from build123d import *

# Parameters (mm, degrees)
SKETCH1_R           = 25
BOSS_EXTRUDE1_DEPTH = 3.5
SKETCH2_R           = 8.05
SKETCH2_R_2         = 6.05
BOSS_EXTRUDE2_DEPTH = 5.5
SKETCH3_R           = 6.15
BOSS_EXTRUDE3_DEPTH = 3


with BuildPart() as part:
    # Sketch1 → Boss-Extrude1 (new body)
    with BuildSketch(Plane(origin=(0, 0, 0), x_dir=(1, 0, 0), z_dir=(0, 1, 0))):
        with Locations(Location((0, 0, 0), (0, 0, 270))):
            Circle(SKETCH1_R)
    extrude(amount=BOSS_EXTRUDE1_DEPTH)

    # Sketch2 → Boss-Extrude2 (add)
    with BuildSketch(Plane(origin=(0, 3.5, 0), x_dir=(1, 0, 0), z_dir=(0, 1, 0))):
        with Locations(Location((0, 0, 0), (0, 0, 270))):
            Circle(SKETCH2_R)
        with Locations(Location((0, 0, 0), (0, 0, 270))):
            Circle(SKETCH2_R_2, mode=Mode.SUBTRACT)
    extrude(amount=BOSS_EXTRUDE2_DEPTH)

    # Sketch3 → Boss-Extrude3 (add)
    with BuildSketch(Plane(origin=(0, 3.5, 0), x_dir=(1, 0, 0), z_dir=(0, 1, 0))):
        Circle(SKETCH3_R)
    extrude(amount=BOSS_EXTRUDE3_DEPTH)


solid = part.part
Source: CAD feature listing. Evaluate the final solid. Frame: model axes, mm. A direction names the side the tool comes from. Round coordinates to 2 decimals unless told otherwise and drop trailing zeros. Order: outer loops, then holes, each group sorted by start corner. A loop starts at its lowest first (then second) coordinate and runs counter-clockwise, first axis right, second up. Notation, with made-up numbers: (68.5, 0.25) - (117.5, 0.25) arc R10 cw to (117.5, 15.25) - close; hole circle Ø4 at (-15.75, -24). An arc over 180 degrees is marked (long way). Use a Markdown table: item, result. Add a question column.
1. Set-up query: faces 1 (the flat face through (6, 3.5, -6)), 2 (the flat face through (0, 0, 0)). Return all of +Z, -Z, +X, -X, +Y, -Y with unobstructed straight access to the full face (end or side cutting, diameter ignored); none if empty.
2. Section query D-D (y = 7.5). Return the cut outline in (x, z), then the cut area to 3 significant figures.
3. Section query B-B (x = 0). Return the cut outline in (y, z).
4. Section query C-C (y = 4.5). Return the cut outline in (x, z), then the cut area to 3 significant figures.
5. First-contact query: pin 1 (5 mm diameter, centred on y = 7, z = -15.5, fed in from +X); pin 2 (5 mm diameter, centred on x = -17, z = 14.5, fed in from +Y); pin 3 (3 mm diameter, centred on x = 17.5, y = 2.5, fed in from +Z); pin 4 (3.5 mm diameter, centred on x = -2, z = 1.5, fed in from +Y). Flat tips, straight axial feed; report the tip coordinate or a pass-through.
6. Mould query, pull axis Z, two halves, no side actions, for faces 3 (the cylindrical face through (7.509, 1.726, 23.846)), 4 (the cylindrical face through (1.82, 7.73, 5.77)), 5 (the flat face through (0, 6.5, 0)), 6 (the flat face through (6, 9, -2)). Classes: +Z half, -Z half, draft (parallel to the pull), parting line (faces both ways), or undercut.
7. Line query: probe 1 along X at (y, z) = (7.5, 0); probe 2 along Y at (x, z) = (16, -5.5); probe 3 along Y at (x, z) = (4, -3). Output: solid intervals per line, ascending.
8. Section query A-A (z = 0). Return the cut outline in (x, y), then the cut area to 3 significant figures.
Derived:
| question | item | result |
|---|---|---|
| 1 | face 1 | +Y |
| 1 | face 2 | +Z, -Z, +X, -X, -Y |
| 2 | outline | circle Ø16.1 at (0, 0); hole circle Ø12.1 at (0, 0) |
| 2 | area | 88.6 mm2 |
| 3 | outline | (0, -25) - (3.5, -25) - (3.5, -8.05) - (9, -8.05) - (9, -6.05) - (6.5, -6.05) - (6.5, 6.05) - (9, 6.05) - (9, 8.05) - (3.5, 8.05) - (3.5, 25) - (0, 25) - close |
| 4 | outline | circle Ø16.1 at (0, 0) |
| 4 | area | 204 mm2 |
| 5 | pin 1 | through |
| 5 | pin 2 | y = 3.5 |
| 5 | pin 3 | z = 19.21 |
| 5 | pin 4 | y = 6.5 |
| 6 | face 3 | parting line |
| 6 | face 4 | undercut |
| 6 | face 5 | undercut |
| 6 | face 6 | draft |
| 7 | probe 1 | -8.05 to -6.05, 6.05 to 8.05 |
| 7 | probe 2 | 0 to 3.5 |
| 7 | probe 3 | 0 to 6.5 |
| 8 | outline | (-25, 0) - (25, 0) - (25, 3.5) - (8.05, 3.5) - (8.05, 9) - (6.05, 9) - (6.05, 6.5) - (-6.05, 6.5) - (-6.05, 9) - (-8.05, 9) - (-8.05, 3.5) - (-25, 3.5) - close |
| 8 | area | 233 mm2 |
